Verification items for the finished model (mm, model axes). Face numbers are marked on the shaded views. A direction names the side the tool comes from. Coordinates: 2 decimals unless noted, no trailing zeros. Order: outer loops, then holes, each group sorted by start corner. A loop starts at its lowest first (then second) coordinate and runs counter-clockwise, first axis right, second up. Notation, with made-up numbers: (72, 37.5) - (96, 37.5) arc R14 ccw to (96, 47.5) - close; hole circle Ø11 at (-35, 59.5). An arc over 180 degrees is marked (long way). Answer as CSV lines item,"result". Start each with the question number.
1. Go/stop test with flat-tipped pins: pin 1 (1.5 mm diameter, centred on x = -11, y = 24, fed in from +Z); pin 2 (20 mm diameter, centred on x = 9, z = 3, fed in from +Y); pin 3 (1 mm diameter, centred on x = 28.5, y = 23.5, fed in from -Z). Record where each tip stops, or that it passes through.
2. Section check B-B (y = 22.5). Record the cut outline in (x, z), and give its area (3 significant figures).
3. Section check C-C (z = 13). Record the cut outline in (x, y).
4. Section check A-A (y = 5). Record the cut outline in (x, z), and give its area (3 significant figures).
5. Mould release check, pull along Z, two halves, no side actions. Record for the marked faces 5, 6 and 7: pulls with the +Z half, pulls with the -Z half, needs draft (parallel to the pull), parting line crosses it, or undercut.
6. Section check D-D (x = 3.5). Record the cut outline in (y, z).
7. Material ranges on L1, parallel to Z at x = -15.5, y = 19.5; L2, parallel to Z at x = 5.5, y = 13, recorded low to high. Write a range as [from, to].
8. Set-up check for the marked faces 1, 2, 3 and 4: record each of +Z, -Z, +X, -X, +Y, -Y from which the full face is reachable in a straight line by a thin tool's end or side.
Autodesk Inventor part; units mm, degrees
ref_plane "YZ Plane" through (0, 0, 0) normal (1, 0, 0) x (0, 1, 0)
ref_plane "XZ Plane" through (0, 0, 0) normal (0, 1, 0) x (-1, 0, 0)
ref_plane "XY Plane" through (0, 0, 0) normal (0, 0, 1) x (1, 0, 0)
sketch "Sketch1" plane through (0, 0, 0) normal (0, 1, 0) x (-1, 0, 0)
  line L0 (-38, 38) -> (38, 38)
  line L1 (38, 38) -> (38, -38)
  line L2 (38, -38) -> (-38, -38)
  line L3 (-38, -38) -> (-38, 38)
  line L4 (-38, 38) -> (38, -38) construction
  line L5 (38, 38) -> (-38, -38) construction
  line L6 (-43.5, 43.5) -> (43.5, 43.5)
  line L7 (43.5, 43.5) -> (43.5, -43.5)
  line L8 (43.5, -43.5) -> (-43.5, -43.5)
  line L9 (-43.5, -43.5) -> (-43.5, 43.5)
  line L10 (-43.5, 43.5) -> (43.5, -43.5) construction
  line L11 (43.5, 43.5) -> (-43.5, -43.5) construction
  point P0 (0, 0)
  dimension "d0" = 76
  dimension "d1" = 76
  dimension "d2" = 87
  dimension "d3" = 87
extrude "Extrusion1" add sketch "Sketch1" along normal blind 36 contours L0 L1 L2 L3
extrude "Extrusion2" add sketch "Sketch1" along normal blind 24 contours L0 L1 L2 L3 | L6 L7 L8 L9
sketch "Sketch2" plane through (0, 36, 0) normal (0, 1, 0) x (1, 0, 0)
  line L0 (33, -33) -> (-33, -33)
  line L1 (-33, -33) -> (-33, 33)
  line L2 (-33, 33) -> (33, 33)
  line L3 (33, 33) -> (33, -33)
  line L4 (33, -33) -> (-33, 33) construction
  line L5 (-33, -33) -> (33, 33) construction
  line L6 (-38, 38) -> (-38, -38)
  line L7 (38, 38) -> (-38, 38)
  point P0 (0, 0)
  dimension "d8" = 5
  dimension "d9" = 5
extrude "Extrusion3" cut sketch "Sketch2" against normal blind 27
fillet "Fillet1" radius 16 12 edges at (38, 30, 38) (38, 30, -38) (-38, 30, -38) (-38, 30, 38) (-43.5, 12, -43.5) (-43.5, 12, 43.5) (43.5, 12, 43.5) (43.5, 12, -43.5) (33, 22.5, 33) (33, 22.5, -33) (-33, 22.5, -33) (-33, 22.5, 33)
ref_plane "Work Plane1" through (0, 0, -27.5) normal (-1, 0, 0) x (0, 0, 1)
move faces "Move1" translate (0, -6, 0) faces at (41.6667, 24, 7.3333)
move faces "Move2" translate (0, -1, 0) faces at (41.6667, 18, -7.3333)
move faces "Move3" translate (0, -5, 0) faces at (5.6667, 36, -36.3333)
properties part number "Podstawka_dla_skurwysyna"
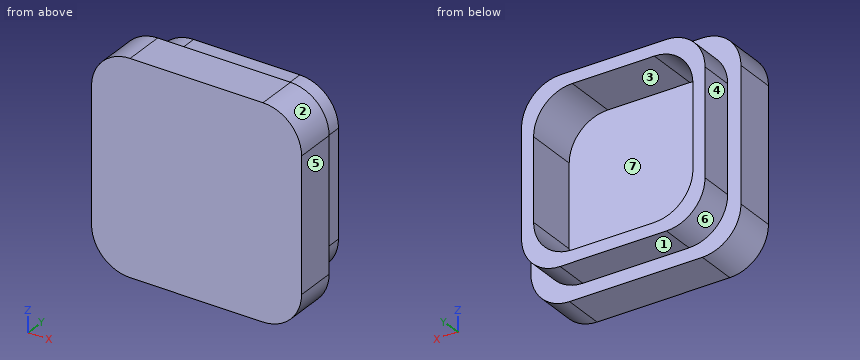
Evaluation:
1,pin 1,"stops at z = 38"
1,pin 2,"stops at y = 9"
1,pin 3,"stops at z = -36.83"
2,outline,"(-38, -22) arc R16 ccw to (-22, -38) - (22, -38) arc R16 ccw to (38, -22) - (38, 22) arc R16 ccw to (22, 38) - (-22, 38) arc R16 ccw to (-38, 22) - close; hole (-33, -17) arc R16 ccw to (-17, -33) - (17, -33) arc R16 ccw to (33, -17) - (33, 17) arc R16 ccw to (17, 33) - (-17, 33) arc R16 ccw to (-33, 17) - close"
2,area,"1,420 mm²"
3,outline,"(-43.5, 0) - (43.5, 0) - (43.5, 17) - (38, 17) - (38, 31) - (33, 31) - (33, 9) - (-33, 9) - (-33, 31) - (-38, 31) - (-38, 17) - (-43.5, 17) - close"
4,outline,"(-43.5, -27.5) arc R16 ccw to (-27.5, -43.5) - (27.5, -43.5) arc R16 ccw to (43.5, -27.5) - (43.5, 27.5) arc R16 ccw to (27.5, 43.5) - (-27.5, 43.5) arc R16 ccw to (-43.5, 27.5) - close"
4,area,"7,350 mm²"
5,face 5,"needs draft"
5,face 6,"pulls with the -Z half"
5,face 7,"undercut"
6,outline,"(0, -43.5) - (17, -43.5) - (17, -38) - (31, -38) - (31, -33) - (9, -33) - (9, 33) - (31, 33) - (31, 38) - (17, 38) - (17, 43.5) - (0, 43.5) - close"
7,L1,"z = [-38, -33], [33, 38]"
7,L2,"z = [-43.5, -33], [33, 43.5]"
8,face 1,"-Z, +X, -X, +Y"
8,face 2,"+Z, +X, +Y, -Y"
8,face 3,"+Y"
8,face 4,"+Z, -Z, -X, +Y"
